from build123d import *

# Parameters (mm, degrees)
SKETCH1_W             = 7
SKETCH1_H             = 5
BOSS_EXTRUDE1_DEPTH   = 20
SKETCH2_W             = 7
SKETCH2_H             = 4
BOSS_EXTRUDE2_DEPTH   = 18
F_3_0MM_DOWEL_HOLE1_D = 3


with BuildPart() as part:
    # Sketch1 → Boss-Extrude1 (new body)
    with BuildSketch(Plane(origin=(0, 0, 0), x_dir=(1, 0, 0), z_dir=(0, 1, 0))):
        Rectangle(SKETCH1_W, SKETCH1_H)
    extrude(amount=BOSS_EXTRUDE1_DEPTH)

    # Sketch2 → Boss-Extrude2 (add)
    with BuildSketch(Plane.XY.offset(2.5)):
        with Locations((0, 18)):
            Rectangle(SKETCH2_W, SKETCH2_H)
    boss_extrude2 = extrude(amount=BOSS_EXTRUDE2_DEPTH)

    # Ø3.0mm Dowel Hole1 (through all)
    with Locations(Plane(origin=(0, 20, 0), x_dir=(1, 0, 0), z_dir=(0, 1, 0))):
        with Locations((0, -15.5)):
            f_3_0mm_dowel_hole1 = Hole(F_3_0MM_DOWEL_HOLE1_D / 2)

    # Mirror1: Boss-Extrude2, Ø3.0mm Dowel Hole1 across plane
    add(boss_extrude2.mirror(Plane.XY))
    add(f_3_0mm_dowel_hole1.mirror(Plane.XY), mode=Mode.SUBTRACT)


solid = part.part
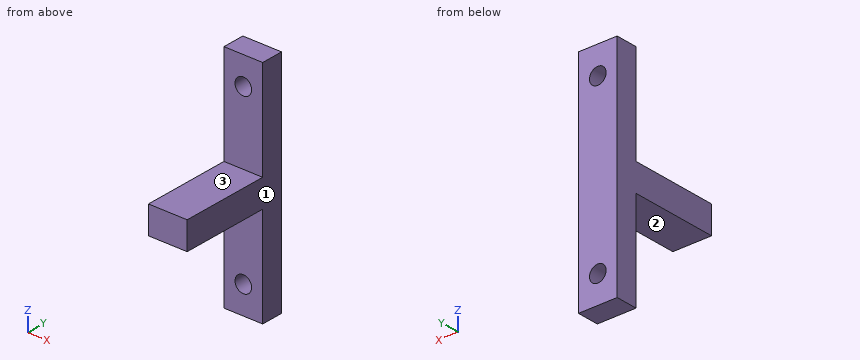
Geometry check sheet. Reference: the model listing, model coordinates, mm. Face numbers are marked on the shaded views. A direction names the side the tool comes from. Round coordinates to 2 decimals unless told otherwise and drop trailing zeros. Loops run counter-clockwise (first coordinate to the right, second up) from the corner with the lowest first, then second, coordinate; pieces in that order, holes last. Notation, with made-up numbers: (12, 38.5) -> (18, 38.5) arc R14 cw to (18, 52.5) -> close; hole circle Ø5 at (59, 26). An arc over 180 degrees is marked (long way). Answer as a JSON object with one key per item and string values. Group by question number.
Item 1: Thickness scan on line 1 along Z through (x, y) = (0, 17.9); line 2 along Z through (x, y) = (1.25, 17.5); line 3 along X through (y, z) = (18.3, 15.5). Record the ranges inside material, lowest first.
Item 2: Cross-section at B-B, the plane z = -15.5. Record the cut outline in (x, y).
Item 3: Cross-section at A-A, the plane x = 0. Record the cut outline in (y, z).
Item 4: Cross-section at D-D, the plane y = 2. Record the cut outline in (x, z), plus the area to 3 significant figures.
Item 5: Depth check by flat-ended pin: pin 1 Ø4 at (x, z) = (0, -15.5) entering from +Y; pin 2 Ø3.5 at (x, z) = (1, -8.5) entering from -Y. Enter the tip coordinate at first touch or a pass-through.
Item 6: Cross-section at C-C, the plane x = -2.5. Record the cut outline in (y, z), plus the area to 3 significant figures.
Item 7: Set-up check for the marked faces 1, 2 and 3: record each of +Z, -Z, +X, -X, +Y, -Y from which the full face is reachable in a straight line by a thin tool's end or side.
Determined:
{
 "1": {"line 1": "z = -20.5 to -17, -14 to 14, 17 to 20.5", "line 2": "z = -20.5 to -16.33, -14.67 to 14.67, 16.33 to 20.5", "line 3": "x = -3.5 to -1.5, 1.5 to 3.5"},
 "2": {"outline": "(-3.5, 16) -> (-1.5, 16) -> (-1.5, 20) -> (-3.5, 20) -> close; (1.5, 16) -> (3.5, 16) -> (3.5, 20) -> (1.5, 20) -> close"},
 "3": {"outline": "(0, -2.5) -> (16, -2.5) -> (16, -14) -> (20, -14) -> (20, 14) -> (16, 14) -> (16, 2.5) -> (0, 2.5) -> close; (16, -20.5) -> (20, -20.5) -> (20, -17) -> (16, -17) -> close; (16, 17) -> (20, 17) -> (20, 20.5) -> (16, 20.5) -> close"},
 "4": {"outline": "(-3.5, -2.5) -> (3.5, -2.5) -> (3.5, 2.5) -> (-3.5, 2.5) -> close", "area": "35.0 mm²"},
 "5": {"pin 1": "stops at y = 20", "pin 2": "stops at y = 16"},
 "6": {"outline": "(0, -2.5) -> (16, -2.5) -> (16, -20.5) -> (20, -20.5) -> (20, 20.5) -> (16, 20.5) -> (16, 2.5) -> (0, 2.5) -> close", "area": "244 mm²"},
 "7": {"face 1": "+Z, -Z, +X, +Y, -Y", "face 2": "-Z, +X, -X, -Y", "face 3": "+Z, +X, -X, -Y"}
}
